Build history of the part. All positions in model axes, mm. A direction names the side the tool comes from. Give positions to 0.01 mm unless a question says otherwise; leave off trailing zeros. Order: outer loops, then holes, each group sorted by start corner. A loop starts at its lowest first (then second) coordinate and runs counter-clockwise, first axis right, second up. Notation, with made-up numbers: (7.5, 85.5) - (55.5, 85.5) arc R24 ccw to (55.5, 102.5) - close; hole circle Ø1 at (81.25, 26). An arc over 180 degrees is marked (long way). Use a Markdown table: item, result. Add a question column.
(1) Which spindle directions (+Z, -Z, +X, -X, +Y, -Y) get a long thin tool onto all of the face, cutting with end or side? Do faces 1 (the face through (-15, 4, 0)), 2 (the face through (0, 2, -22)), 3 (the face through (19.5, 1, 0)). Say none if no direction does.
(2) Mould opens along Z. For faces 4 (the face through (0, 2, 22)), 5 (the face through (15, 4, 0)), 6 (the face through (0, 1, 19.5)), 7 (the face through (-20, 0, -3)) say: +Z half, -Z half, draft (parallel to the pull), parting line (faces both ways), or undercut.
(3) Slice it at A-A (z = 11.5). Write the cut outline in (x, y).
(4) Wall check: line 1 (Z direction, x = 10, y = 4.2); line 2 (X direction, y = 0.8, z = -13.5). Give the ranges that are in metal, low to high.
(5) Slice it at C-C (x = 11.5). Write the cut outline in (y, z), then the cut area to 3 significant figures.
(6) Flat gauge pin, fed straight in: pin 1 (6 mm diameter, centred on x = 9.5, z = -10, fed in from +Y). Where does the tip first touch, or does it go through?
(7) Slice it at B-B (y = 4.5). Write the cut outline in (x, z).
from build123d import *

# Parameters (mm, degrees)
SKETCH1_W           = 44
SKETCH1_H           = 44
BOSS_EXTRUDE1_DEPTH = 5
SKETCH3_W           = 30
SKETCH3_H           = 30
CUT_EXTRUDE1_DEPTH  = 2
SKETCH5_W           = 39
SKETCH5_H           = 39
CUT_EXTRUDE3_DEPTH  = 3


with BuildPart() as part:
    # Sketch1 → Boss-Extrude1 (new body)
    with BuildSketch(Plane(origin=(0, 0, 0), x_dir=(1, 0, 0), z_dir=(0, 1, 0))):
        Rectangle(SKETCH1_W, SKETCH1_H)
    extrude(amount=BOSS_EXTRUDE1_DEPTH)

    # Sketch3 → Cut-Extrude1 (cut)
    with BuildSketch(Plane(origin=(0, 5, 0), x_dir=(1, 0, 0), z_dir=(0, 1, 0))):
        Rectangle(SKETCH3_W, SKETCH3_H)
    extrude(amount=-CUT_EXTRUDE1_DEPTH, mode=Mode.SUBTRACT)

    # Sketch5 → Cut-Extrude3 (cut)
    with BuildSketch(Plane.XZ):
        Rectangle(SKETCH5_W, SKETCH5_H)
    extrude(amount=-CUT_EXTRUDE3_DEPTH, mode=Mode.SUBTRACT)


solid = part.part
Solution:
| question | item | result |
|---|---|---|
| 1 | face 1 | +Y, -Y |
| 1 | face 2 | -Z, +X, -X, +Y, -Y |
| 1 | face 3 | -Y |
| 2 | face 4 | +Z half |
| 2 | face 5 | undercut |
| 2 | face 6 | undercut |
| 2 | face 7 | draft |
| 3 | outline | (-22, 0) - (-19.5, 0) - (-19.5, 3) - (-15, 3) - (-15, 5) - (-22, 5) - close; (15, 3) - (19.5, 3) - (19.5, 0) - (22, 0) - (22, 5) - (15, 5) - close |
| 4 | line 1 | -22 to -15, 15 to 22 |
| 4 | line 2 | -22 to -19.5, 19.5 to 22 |
| 5 | outline | (0, -22) - (5, -22) - (5, -15) - (3, -15) - (3, -19.5) - (0, -19.5) - close; (0, 19.5) - (3, 19.5) - (3, 15) - (5, 15) - (5, 22) - (0, 22) - close |
| 5 | area | 43.0 mm2 |
| 6 | pin 1 | through |
| 7 | outline | (-22, -22) - (22, -22) - (22, 22) - (-22, 22) - close; hole (-15, -15) - (15, -15) - (15, 15) - (-15, 15) - close |
